The model under review builds one solid part; all positions refer to its coordinate system, in mm. A direction names the side the tool comes from. Round coordinates to 2 decimals unless told otherwise and drop trailing zeros. Write item = value, one per line. Start each with the question number.
Item 1: The part is to be moulded in two halves that separate along Z. For faces 4 (the cylindrical face through (-8.88, -4.87, 21.78)), 5 (the flat face through (-11.6, -12.7, 8.7)), 6 (the flat face through (10.8, -11.2, 11.4)), say which applies: +Z half, -Z half, draft (parallel to the pull), parting line (faces both ways), or undercut.
Item 2: For pin 1 Ø10 at (y, z) = (-5.5, 4) entering from -X; pin 2 Ø1.5 at (x, y) = (-6.5, 9) entering from -Z; pin 3 Ø1.5 at (y, z) = (3.5, 22.5) entering from -X, all flat-tipped, find the tip position at first contact; note any pin that passes through.
Item 3: Tool access review of faces 1 (the flat face through (-9.882, -11.166, 6.019)), 2 (the flat face through (-1.3, -11.2, 9.7)), 3 (the flat face through (11.6, -12.7, 8.7)): name each direction out of +Z, -Z, +X, -X, +Y, -Y from which nothing blocks a thin tool from reaching the whole face with its end or side.
Item 4: To check wall thickness, follow line 1 along Z through (x, y) = (-4.75, -10.5); line 2 along Z through (x, y) = (-6, -11); line 3 along Z through (x, y) = (2, 0). State the ranges of each line that lie inside material, in increasing order.
Autodesk Inventor part; units mm, degrees
ref_plane "YZ Plane" through (0, 0, 0) normal (1, 0, 0) x (0, 1, 0)
ref_plane "XZ Plane" through (0, 0, 0) normal (0, 1, 0) x (-1, 0, 0)
ref_plane "XY Plane" through (0, 0, 0) normal (0, 0, 1) x (1, 0, 0)
sketch "Sketch1" plane through (0, 0, 0) normal (0, 0, 1) x (1, 0, 0)
  arc A0 (12.7, 3.175) -> (-12.7, 3.175) centre (0, 3.175) ccw
  line L0 (-12.7, 3.175) -> (-12.7, -12.7)
  line L1 (-12.7, -12.7) -> (12.7, -12.7)
  line L2 (12.7, -12.7) -> (12.7, 3.175)
  line L3 (-12.7, -12.7) -> (-11.1125, -12.7)
  line L4 (-11.1125, -12.7) -> (-7.9375, -12.7)
  line L5 (-7.9375, -12.7) -> (-7.9375, -10.16)
  line L6 (-7.9375, -10.16) -> (-11.1125, -12.7)
  line L7 (-7.9375, -10.16) -> (-4.7625, -12.7)
  line L8 (12.7, -12.7) -> (11.1125, -12.7)
  line L9 (11.1125, -12.7) -> (7.9375, -12.7)
  line L10 (7.9375, -12.7) -> (7.9375, -10.16)
  line L11 (7.9375, -10.16) -> (11.1125, -12.7)
  line L12 (7.9375, -12.7) -> (4.7625, -12.7)
  line L13 (4.7625, -12.7) -> (7.9375, -10.16)
  line L14 (0, -12.7) -> (0, -10.16)
  line L15 (0, -12.7) -> (3.175, -12.7)
  line L16 (3.175, -12.7) -> (0, -10.16)
  line L17 (0, -12.7) -> (-3.175, -12.7)
  line L18 (-3.175, -12.7) -> (0, -10.16)
  dimension "d5" = 25.4
  dimension "d6" = 15.875
  dimension "d7" = 25.4
  dimension "d8" = 1.5875
  dimension "d9" = 3.175
  dimension "d10" = 2.54
  dimension "d11" = 3.175
  dimension "d12" = 1.5875
  dimension "d13" = 3.175
  dimension "d14" = 2.54
  dimension "d15" = 3.175
  dimension "d16" = 2.54
  dimension "d17" = 3.175
  dimension "d18" = 3.175
extrude "Extrusion1" add sketch "Sketch1" along normal blind 25.4 contours L2 L1 L11 L13 L16 L18 L7 L6 L0 A0
fillet "Fillet1" radius 12.7 6 edges at (-12.7, -4.7625, 25.4) (12.7, -4.7625, 25.4) (0, 15.875, 25.4) (-12.7, -4.7625, 0) (12.7, -4.7625, 0) (0, 15.875, 0)
sketch "Sketch2" plane through (0, 0, 0) normal (1, 0, 0) x (0, 1, 0)
  arc A0 (3.1749, 0) -> (3.1749, 25.4) centre (3.1749, 12.7) ccw
  line L0 (3.1749, 25.4) -> (-12.7001, 25.4)
  line L1 (-12.7001, 25.4) -> (-12.7001, 0)
  line L2 (-12.7001, 0) -> (3.1749, 0)
  line L3 (-12.7001, 25.4) -> (-12.7001, 23.8125)
  line L4 (-12.7001, 23.8125) -> (-12.7001, 20.6375)
  line L5 (-12.7001, 20.6375) -> (-10.1601, 20.6375)
  line L6 (-10.1601, 20.6375) -> (-12.7001, 23.8125)
  line L7 (-10.1601, 20.6375) -> (-12.7001, 17.4625)
  line L8 (-12.7001, 0) -> (-12.7001, 1.5875)
  line L9 (-12.7001, 1.5875) -> (-12.7001, 4.7625)
  line L10 (-12.7001, 4.7625) -> (-10.1601, 4.7625)
  line L11 (-10.1601, 4.7625) -> (-12.7001, 1.5875)
  line L12 (-12.7001, 4.7625) -> (-12.7001, 7.9375)
  line L13 (-12.7001, 7.9375) -> (-10.1601, 4.7625)
  line L14 (-12.7001, 12.7) -> (-10.1601, 12.7)
  line L15 (-12.7001, 12.7) -> (-12.7001, 9.525)
  line L16 (-12.7001, 9.525) -> (-10.1601, 12.7)
  line L17 (-12.7001, 12.7) -> (-12.7001, 15.875)
  line L18 (-12.7001, 15.875) -> (-10.1601, 12.7)
  line L19 (3.175, 25.4) -> (3.175, 0)
  point P0 (0, 0)
  dimension "d22" = 25.4
  dimension "d23" = 15.875
  dimension "d24" = 25.4
  dimension "d25" = 1.5875
  dimension "d26" = 3.175
  dimension "d27" = 2.54
  dimension "d28" = 3.175
  dimension "d29" = 1.5875
  dimension "d30" = 3.175
  dimension "d31" = 2.54
  dimension "d32" = 3.175
  dimension "d33" = 2.54
  dimension "d34" = 3.175
  dimension "d35" = 3.175
extrude "Extrusion2" cut sketch "Sketch2" along normal mid plane 25.4 contours L19 A0 | L2 L1 L11 L13 L16 L18 L7 L6 L0 L19 keep common part
equation "\"d6\" = 0.625 * d5"
equation "\"d7\" = d5"
equation "\"d8\" = 0.0625 * d7"
equation "\"d9\" = 0.125 * d7"
equation "\"d11\" = d9"
equation "\"d12\" = d8"
equation "\"d13\" = d9"
equation "\"d14\" = d10"
equation "\"d15\" = d9"
equation "\"d16\" = d10"
equation "\"d17\" = d9"
equation "\"d18\" = d9"
equation "\"d23\" = 0.625 * d22"
equation "\"d24\" = d22"
equation "\"d25\" = 0.0625 * d24"
equation "\"d26\" = 0.125 * d24"
equation "\"d28\" = d26"
equation "\"d29\" = d25"
equation "\"d30\" = d26"
equation "\"d31\" = d27"
equation "\"d32\" = d26"
equation "\"d33\" = d27"
equation "\"d34\" = d26"
equation "\"d35\" = d26"
properties part number "Ghost1"
Response values:
q1.face_4 = +Z half
q1.face_5 = draft
q1.face_6 = undercut
q2.pin_1 = -12.15
q2.pin_2 = 2.82
q2.pin_3 = -8.9
q3.face_1 = +X, -X, -Y
q3.face_2 = +Z, -Z, -Y
q3.face_3 = +Z, -Z, +X, -X, -Y
q4.line_1 = 0.92 to 4.34, 5.19 to 12.28, 13.12 to 20.21, 21.06 to 24.48
q4.line_2 = 1.51 to 3.71, 5.81 to 11.65, 13.75 to 19.59, 21.69 to 23.89
q4.line_3 = 0.16 to 25.24
